Source: three-view drawing plus pictorial views. Frame: mm from the lowest corner of the part. A direction names the side the tool comes from. Give positions to 0.01 mm unless a question says otherwise; leave off trailing zeros. Write each loop counter-clockwise with the first axis right and the second up, starting at its lowest first coordinate (ties: lowest second). Pieces come first, ordered by that corner, then holes. Notation, with made-up numbers: M 22,-29 L 65,-29 A24 cw 65,-7 Z; hole C 21.25,-3 d1. An arc over 180 degrees is marked long. Return JSON: item names as keys, results as strings.
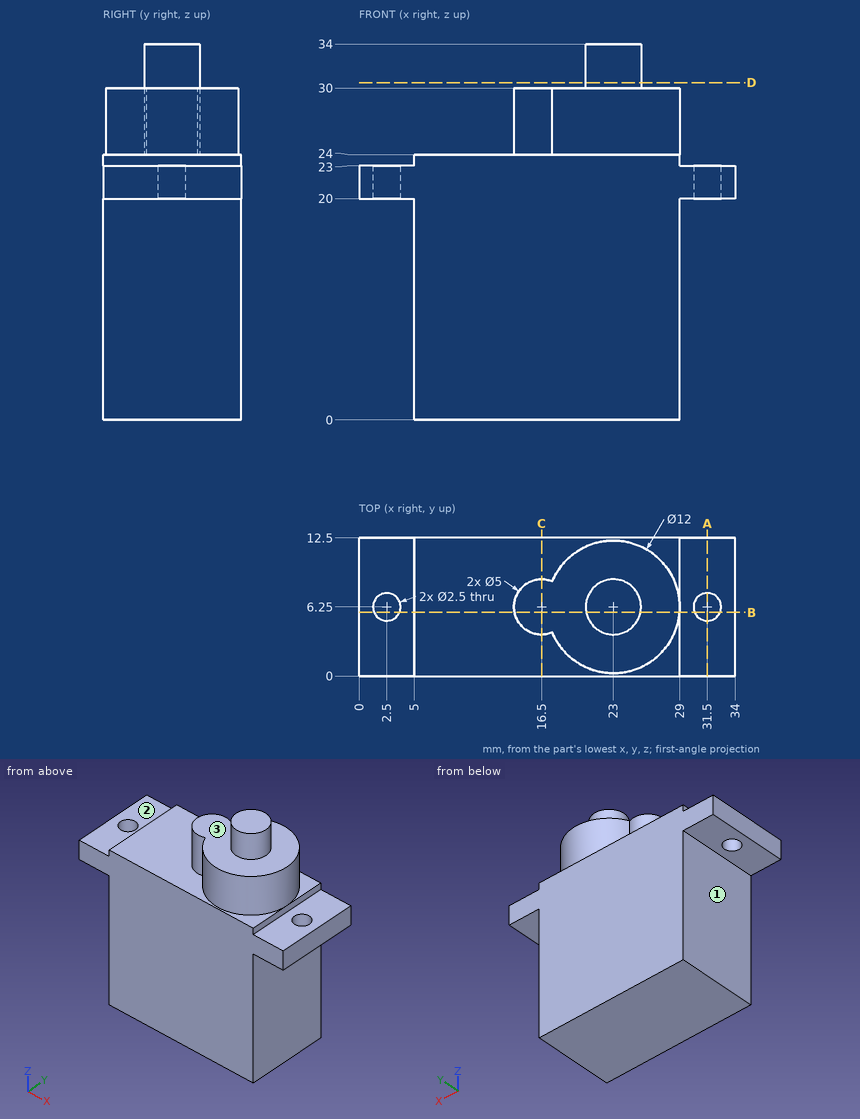
1) Cut plane D-D, the plane z = 30.5. Return the cut outline in (x, y), then the cut area to 3 significant figures.
Numbers:
{"outline": "C 23,6.25 d5", "area": "19.6 mm²"}
2) Cut plane C-C, the plane x = 16.5. Return the cut outline in (y, z).
Numbers:
{"outline": "M 0,0 L 12.5,0 L 12.5,24 L 8.75,24 L 8.75,30 L 3.75,30 L 3.75,24 L 0,24 Z"}
3) Cut plane A-A, the plane x = 31.5. Return the cut outline in (y, z).
Numbers:
{"outline": "M 0,20 L 5,20 L 5,23 L 0,23 Z; M 7.5,20 L 12.5,20 L 12.5,23 L 7.5,23 Z"}
4) Set-up query: the marked faces 1, 2 and 3. Return all of +Z, -Z, +X, -X, +Y, -Y with unobstructed straight access to the full face (end or side cutting, diameter ignored); none if empty.
Numbers:
{"face 1": "-Z, -X, +Y, -Y", "face 2": "+Z, -X, +Y, -Y", "face 3": "+Z"}
5) Line query: line 1 (X direction, y = 6.25, z = 21.7); line 2 (Y direction, x = 2.5, z = 22); line 3 (X direction, y = 9, z = 15). Output: solid intervals per line, ascending. Write a range as [from, to].
Numbers:
{"line 1": "x = [0, 1.25], [3.75, 30.25], [32.75, 34]", "line 2": "y = [0, 5], [7.5, 12.5]", "line 3": "x = [5, 29]"}
6) Cut plane B-B, the plane y = 5.75. Give the number of separate pieces and of enclosed holes in the cut face, then the cut area to 3 significant figures.
Numbers:
{"separate pieces": "3", "enclosed holes": "0", "area": "701 mm²"}
7) Contact query for flat-ended pins moving along their axis: pin 1 Ø2 at (x, y) = (19, 11) entering from +Z; pin 2 Ø4 at (x, y) = (32, 6.5) entering from +Z; pin 3 Ø6 at (y, z) = (9, 10.5) entering from -X. Output: stop coordinate, or through.
Numbers:
{"pin 1": "stops at z = 30", "pin 2": "stops at z = 23", "pin 3": "stops at x = 5"}
